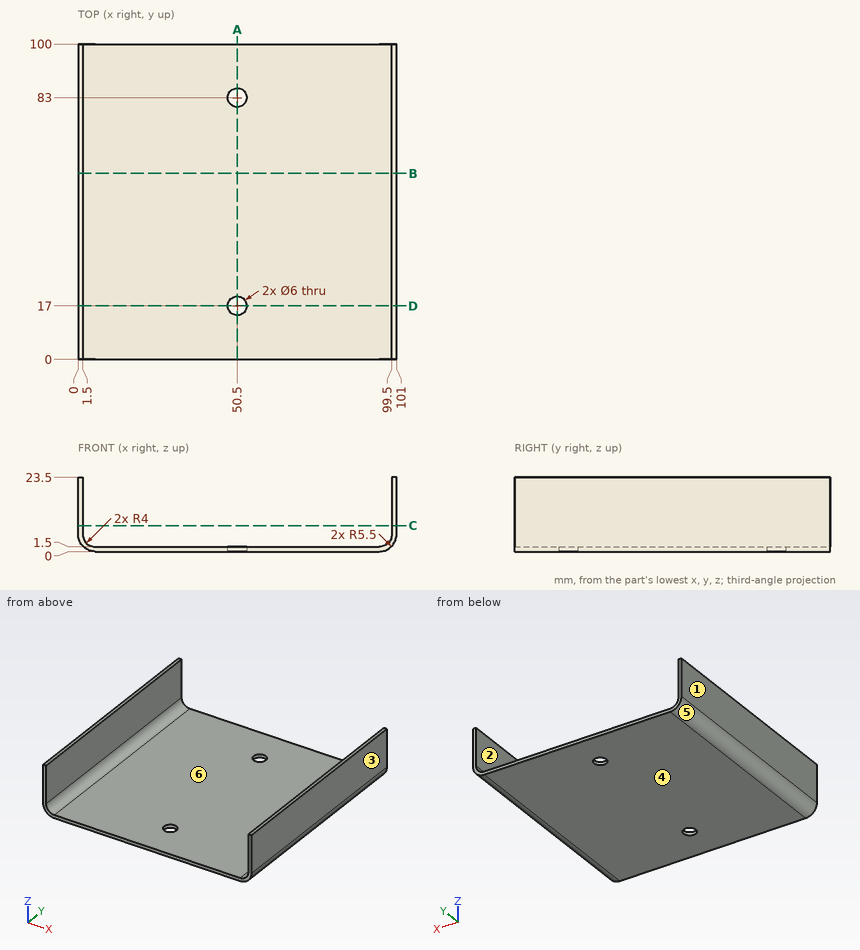
Verification items for this drawing (mm, ordinates from the low corner). A direction names the side the tool comes from. Give positions to 0.01 mm unless a question says otherwise; leave off trailing zeros. Write each loop counter-clockwise with the first axis right and the second up, starting at its lowest first coordinate (ties: lowest second). Pieces come first, ordered by that corner, then holes. Notation, with made-up numbers: (5, 78) -> (35, 78) arc R31 ccw to (35, 114) -> close; hole circle Ø9 at (51, 61). An arc over 180 degrees is marked (long way). Use CSV: the item, a comma, the result in double quotes. Start each with the question number.
Q1. Release check for a two-part mould opening along X. For the marked faces 3, 4, 5 and 6 record: +X half, -X half, draft (parallel to the pull), parting line (faces both ways), or undercut.
Q2. Cross-section at D-D on y = 17. Enter the section's corners in (x, z), and give its area (3 significant figures).
Q3. Cross-section at C-C on z = 8.25. Enter the section's corners in (x, y).
Q4. Cross-section at B-B on y = 59. Enter the section's corners in (x, z), and give its area (3 significant figures).
Q5. Depth check by flat-ended pin: P1, Ø10, axis at x = 55, y = 50, coming from the +Z side; P2, Ø3.5, axis at x = 50.5, y = 17, coming from the -Z side. Enter the tip coordinate at first touch or a pass-through.
Q6. Cross-section at A-A on x = 50.5. Enter the section's corners in (y, z), and give its area (3 significant figures).
Q7. Scan lines: line 1 along Y through (x, z) = (50.5, 0.4); line 2 along X through (y, z) = (76.5, 8.25); line 3 along Z through (x, y) = (38.5, 61). Record each from-to range of solid material in increasing order.
Q8. Tool access check on the marked faces 1 and 2. Record the directions out of +Z, -Z, +X, -X, +Y, -Y that give a thin tool (end or side, any length) a straight path to the whole face; none if there is none.
Working result:
1,face 3,"+X half"
1,face 4,"draft"
1,face 5,"-X half"
1,face 6,"undercut"
2,outline,"(0, 5.5) arc R5.5 ccw to (5.5, 0) -> (47.5, 0) -> (47.5, 1.5) -> (5.5, 1.5) arc R4 cw to (1.5, 5.5) -> (1.5, 23.5) -> (0, 23.5) -> close; (53.5, 0) -> (95.5, 0) arc R5.5 ccw to (101, 5.5) -> (101, 23.5) -> (99.5, 23.5) -> (99.5, 5.5) arc R4 cw to (95.5, 1.5) -> (53.5, 1.5) -> close"
2,area,"202 mm^2"
3,outline,"(0, 0) -> (1.5, 0) -> (1.5, 100) -> (0, 100) -> close; (99.5, 0) -> (101, 0) -> (101, 100) -> (99.5, 100) -> close"
4,outline,"(0, 5.5) arc R5.5 ccw to (5.5, 0) -> (95.5, 0) arc R5.5 ccw to (101, 5.5) -> (101, 23.5) -> (99.5, 23.5) -> (99.5, 5.5) arc R4 cw to (95.5, 1.5) -> (5.5, 1.5) arc R4 cw to (1.5, 5.5) -> (1.5, 23.5) -> (0, 23.5) -> close"
4,area,"211 mm^2"
5,P1,"stops at z = 1.5"
5,P2,"passes through"
6,outline,"(0, 0) -> (14, 0) -> (14, 1.5) -> (0, 1.5) -> close; (20, 0) -> (80, 0) -> (80, 1.5) -> (20, 1.5) -> close; (86, 0) -> (100, 0) -> (100, 1.5) -> (86, 1.5) -> close"
6,area,"132 mm^2"
7,line 1,"y = 0 to 14, 20 to 80, 86 to 100"
7,line 2,"x = 0 to 1.5, 99.5 to 101"
7,line 3,"z = 0 to 1.5"
8,face 1,"+Z, -Z, -X, +Y, -Y"
8,face 2,"+Z, +Y, -Y"
